The drawing under review shows one solid part. Ordinate dimensions are in mm from its lowest x, y, z. A direction names the side the tool comes from. Coordinates: 2 decimals unless noted, no trailing zeros. Loops run counter-clockwise (first coordinate to the right, second up) from the corner with the lowest first, then second, coordinate; pieces in that order, holes last. Notation, with made-up numbers: M -36,30 L -17,30 A22 ccw -17,66 Z; hole C 14.5,-7 d10. An arc over 180 degrees is marked long. Return JSON: item names as keys, results as strings.
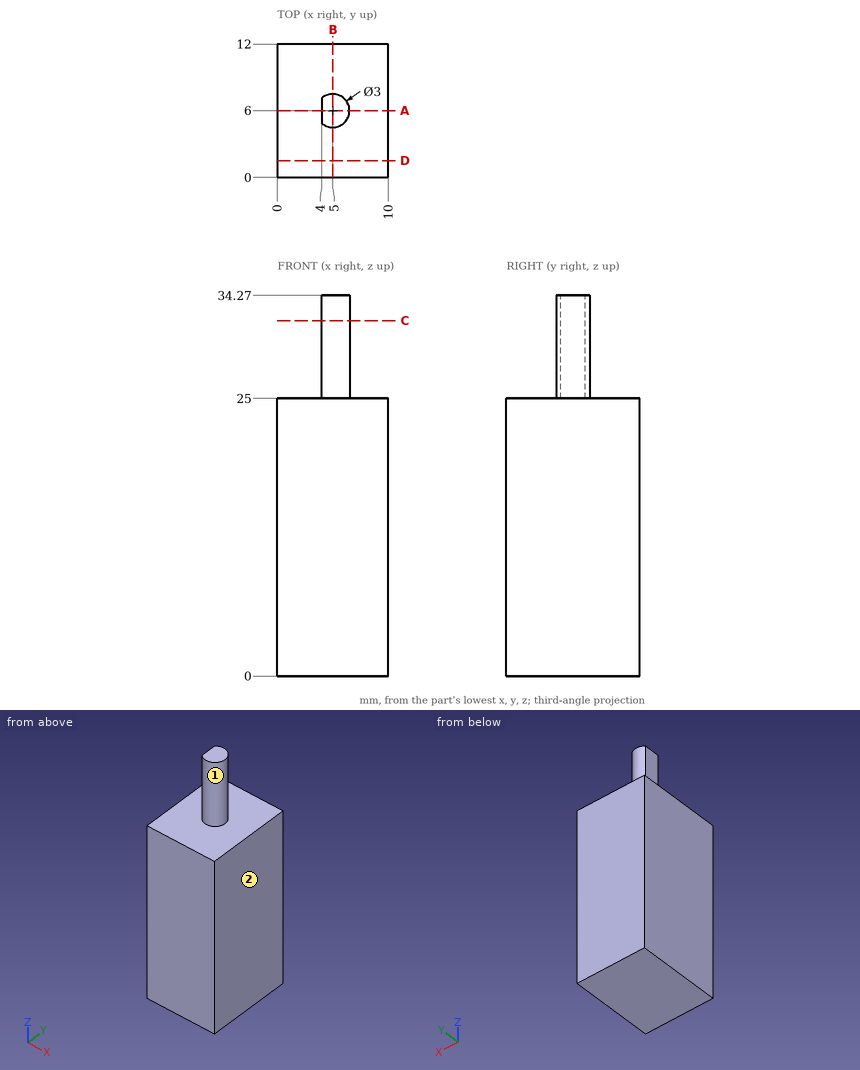
1. Add section D-D on y = 1.5. Give the boundary of the cut face in (x, z).
Check values:
{"outline": "M 0,0 L 10,0 L 10,25 L 0,25 Z"}
2. Add section A-A on y = 6. Give the boundary of the cut face in (x, z).
Check values:
{"outline": "M 0,0 L 10,0 L 10,25 L 6.5,25 L 6.5,34.27 L 4,34.27 L 4,25 L 0,25 Z"}
3. Machinability: for the marked faces 1 and 2, which of the approach directions +Z, -Z, +X, -X, +Y, -Y give a long, thin tool a straight path to every point of the face, cutting with its end or side? Answer none if there is none.
Check values:
{"face 1": "+Z", "face 2": "+Z, -Z, +X, +Y, -Y"}
4. Insertion check: pin 1 Ø6 at (x, y) = (2.5, 2) entering from +Z; pin 2 Ø2.5 at (y, z) = (6, 30.5) entering from -X. Each pin has a flat end and moves straight along its axis. Give the tip position at first contact, or say it passes through.
Check values:
{"pin 1": "z = 25", "pin 2": "x = 4"}
5. To check wall thickness, follow line 1 (Z direction, x = 7, y = 10); line 2 (Y direction, x = 5, z = 30.5); line 3 (X direction, y = 6.5, z = 29). State the ranges of each line that lie inside material, in increasing order.
Check values:
{"line 1": "0 to 25", "line 2": "4.5 to 7.5", "line 3": "4 to 6.41"}
6. Add section B-B on x = 5. Give the boundary of the cut face in (y, z), plus the area to 3 significant figures.
Check values:
{"outline": "M 0,0 L 12,0 L 12,25 L 7.5,25 L 7.5,34.27 L 4.5,34.27 L 4.5,25 L 0,25 Z", "area": "328 mm²"}
7. Add section C-C on z = 32. Give the boundary of the cut face in (x, y), plus the area to 3 significant figures.
Check values:
{"outline": "M 4,4.88 A1.5 ccw long 4,7.12 Z", "area": "6.29 mm²"}
